from build123d import *

# Parameters (mm, degrees)
CHAMFER_SIZE    = 0.5
CHAMFER001_SIZE = 0.5
SKETCH001_W     = 70
SKETCH001_H     = 70
SKETCH001_W_2   = 27.7
SKETCH001_H_2   = 22
POCKET_DEPTH    = 5.001
SKETCH002_W     = 8
SKETCH002_H     = 22
PAD_DEPTH       = 12.1
SKETCH003_W     = 8
SKETCH003_H     = 14.2
POCKET001_DEPTH = 4.6
SKETCH004_W     = 8
SKETCH004_H     = 10
POCKET002_DEPTH = 1.4
SKETCH005_R     = 1.25
POCKET003_DEPTH = 10
FILLET_R        = 10.999
FILLET001_R     = 10.999
FILLET002_R     = 3.999
FILLET003_R     = 3.999
FILLET004_R     = 3.999
FILLET005_R     = 3.999
CHAMFER002_SIZE = 0.5
SKETCH006_W     = 10
SKETCH006_H     = 1
POCKET004_DEPTH = 6
CHAMFER003_SIZE = 0.3
CHAMFER004_SIZE = 0.3


with BuildPart() as part:
    # Sketch → Revolution (revolve)
    with BuildSketch(Plane.XY):
        with BuildLine():
            Line((7.704544, 2.5), (31, 2.5))
            Line((31, 2.5), (31, -2.5))
            Line((7.704544, -2.5), (31, -2.5))
            ThreePointArc((7.704544, -2.5), (7.891937, -1.824097), (8.020154, -1.134517))
            ThreePointArc((8.020154, -1.134517), (8.748074, 0), (8.020154, 1.134517))
            ThreePointArc((8.020154, 1.134517), (7.891937, 1.824097), (7.704544, 2.5))
        make_face()
    revolve(axis=Axis((0, 0, 0), (0, 1, 0)))

    # Chamfer
    chamfer_edges = [part.edges().sort_by_distance(p)[0] for p in [
        (-7.704544, -2.5, 0),
    ]]
    chamfer(chamfer_edges, length=CHAMFER_SIZE)

    # Chamfer001
    chamfer001_edges = [part.edges().sort_by_distance(p)[0] for p in [
        (-7.704544, 2.5, 0),
    ]]
    chamfer(chamfer001_edges, length=CHAMFER001_SIZE)

    # Sketch001 → Pocket (cut, through all)
    with BuildSketch(Plane.XZ.offset(2.5)):
        Rectangle(SKETCH001_W, SKETCH001_H)
        with Locations((2.85, 0)):
            Rectangle(SKETCH001_W_2, SKETCH001_H_2, mode=Mode.SUBTRACT)
    extrude(amount=-POCKET_DEPTH, mode=Mode.SUBTRACT)

    # Sketch002 → Pad (new body)
    with BuildSketch(Plane.XZ.offset(2.5)):
        with Locations((12.7, 0)):
            Rectangle(SKETCH002_W, SKETCH002_H)
    extrude(amount=PAD_DEPTH)

    # Sketch003 → Pocket001 (cut)
    with BuildSketch(Plane.XZ.offset(14.6)):
        with Locations((12.7, 0)):
            Rectangle(SKETCH003_W, SKETCH003_H)
    extrude(amount=-POCKET001_DEPTH, mode=Mode.SUBTRACT)

    # Sketch004 → Pocket002 (cut)
    with BuildSketch(Plane.XZ.offset(10)):
        with Locations((12.7, 0)):
            Rectangle(SKETCH004_W, SKETCH004_H)
    extrude(amount=-POCKET002_DEPTH, mode=Mode.SUBTRACT)

    # Sketch005 → Pocket003 (cut)
    with BuildSketch(Plane.XZ.offset(8.6)):
        with Locations((11.7, 0)):
            Circle(SKETCH005_R)
    extrude(amount=-POCKET003_DEPTH, mode=Mode.SUBTRACT)

    # Fillet
    fillet_edges = [part.edges().sort_by_distance(p)[0] for p in [
        (-11, 0, 11),
    ]]
    fillet(fillet_edges, radius=FILLET_R)

    # Fillet001
    fillet001_edges = [part.edges().sort_by_distance(p)[0] for p in [
        (-11, 0, -11),
    ]]
    fillet(fillet001_edges, radius=FILLET001_R)

    # Fillet002
    fillet002_edges = [part.edges().sort_by_distance(p)[0] for p in [
        (8.7, -8.55, -11),
    ]]
    fillet(fillet002_edges, radius=FILLET002_R)

    # Fillet003
    fillet003_edges = [part.edges().sort_by_distance(p)[0] for p in [
        (16.7, -8.55, -11),
    ]]
    fillet(fillet003_edges, radius=FILLET003_R)

    # Fillet004
    fillet004_edges = [part.edges().sort_by_distance(p)[0] for p in [
        (8.7, -8.55, 11),
    ]]
    fillet(fillet004_edges, radius=FILLET004_R)

    # Fillet005
    fillet005_edges = [part.edges().sort_by_distance(p)[0] for p in [
        (16.7, -8.55, 11),
    ]]
    fillet(fillet005_edges, radius=FILLET005_R)

    # Chamfer002
    chamfer002_edges = [part.edges().sort_by_distance(p)[0] for p in [
        (16.7, 2.5, 0),
    ]]
    chamfer(chamfer002_edges, length=CHAMFER002_SIZE)

    # Sketch006 → Pocket004 (cut)
    with BuildSketch(Plane.XZ.offset(2.5)):
        with Locations((-10, 0)):
            Rectangle(SKETCH006_W, SKETCH006_H)
    extrude(amount=-POCKET004_DEPTH, mode=Mode.SUBTRACT)

    # Chamfer003
    chamfer003_edges = [part.edges().sort_by_distance(p)[0] for p in [
        (-9.338714, 2.5, -0.5),
    ]]
    chamfer(chamfer003_edges, length=CHAMFER003_SIZE)

    # Chamfer004
    chamfer004_edges = [part.edges().sort_by_distance(p)[0] for p in [
        (-9.338714, 2.5, 0.5),
    ]]
    chamfer(chamfer004_edges, length=CHAMFER004_SIZE)


solid = part.part
Read the model definition and answer for the solid it produces. Units are mm, in the model's axes. A direction names the side the tool comes from. Give positions to 0.01 mm unless a question says otherwise; leave off trailing zeros. Write each loop counter-clockwise with the first axis right and the second up, starting at its lowest first coordinate (ties: lowest second). Pieces come first, ordered by that corner, then holes. Notation, with made-up numbers: (43, -16.5) -> (59, -16.5) arc R28 ccw to (59, 21.5) -> close; hole circle Ø6 at (77.5, -0.5). An arc over 180 degrees is marked (long way). Answer as a JSON object with one key per item and string values. Group by question number.
1) A tool of negligible diameter and unlimited length cuts with its end or side. For faces 4 (the flat face through (12, 1.4, 0)), 5 (the flat face through (14, -8.6, 0)), 6 (the cylindrical face through (9.903, -8.635, -9.86)), 7 (the flat face through (8.7, -5, 0)), 8 (the flat face through (-9, 0, 0.5)), from which of +Z, -Z, +X, -X, +Y, -Y can it reach the whole face along a straight path? Write none if from no direction.
2) Consider L1, parallel to Y at x = -3.25, z = -9.5; L2, parallel to Y at x = 12, z = 5.75; L3, parallel to X at y = -3.25, z = 3.5. Determine where each line is inside the solid, lowest interval first. Write a range as from..to.
3) Find section A-A (y = 0). Write down the section's boundary in (x, z).
4) Find section B-B (x = 11.7). Write down the section's boundary in (y, z).
5) The mould has two halves that part along Z. Classify faces 1 (the flat face through (13, -10, -6)), 2 (the flat face through (9, 2.5, 0)), 3 (the cylindrical face through (9.903, -8.635, 9.86)): +Z half, -Z half, draft (parallel to the pull), parting line (faces both ways), or undercut.
6) Each of these flat-tipped pins is pushed along its axis until it touches: P1, Ø1.5, axis at x = 11, y = -9.5, coming from the +Z side; P2, Ø3.5, axis at x = -9.5, y = 0.5, coming from the +Z side; P3, Ø0.8, axis at x = 11.5, z = 0.5, coming from the -Y side; P4, Ø2.5, axis at x = 11, z = 6.5, coming from the -Y side. Where does it stop, or does it pass through?
Values follow:
{
 "1": {"face 4": "-Y", "face 5": "+X, -X, -Y", "face 6": "-Z, -X, -Y", "face 7": "+Z, -Z, -X, -Y", "face 8": "-X, +Y, -Y"},
 "2": {"L1": "y = -2.5..2.5", "L2": "y = -10..2.5", "L3": "x = 8.7..16.7"},
 "3": {"outline": "(-10.99, -0.5) arc R11 ccw to (0, -11) -> (12.7, -11) arc R4 ccw to (16.7, -7) -> (16.7, 7) arc R4 ccw to (12.7, 11) -> (0, 11) arc R11 ccw to (-10.99, 0.5) -> (-8.73, 0.5) arc R8.75 cw (long way) to (-8.73, -0.5) -> close; hole circle Ø2.5 at (11.7, 0)"},
 "4": {"outline": "(-14.6, -10.87) -> (-2.5, -10.87) -> (-2.5, -11) -> (2, -11) -> (2.5, -10.5) -> (2.5, 10.5) -> (2, 11) -> (-2.5, 11) -> (-2.5, 10.87) -> (-14.6, 10.87) -> (-14.6, 7.1) -> (-10, 7.1) -> (-10, 5) -> (-8.6, 5) -> (-8.6, 1.25) -> (1.4, 1.25) -> (1.4, -1.25) -> (-8.6, -1.25) -> (-8.6, -5) -> (-10, -5) -> (-10, -7.1) -> (-14.6, -7.1) -> close"},
 "5": {"face 1": "undercut", "face 2": "draft", "face 3": "+Z half"},
 "6": {"P1": "stops at z = 10.89", "P2": "stops at z = 7.81", "P3": "stops at y = 1.4", "P4": "stops at y = -14.6"}
}
